Design review of the part built by this model. Coordinates are the model's own, in mm. Face numbers are marked on the shaded views. Coordinates: 2 decimals unless noted, no trailing zeros. Write each loop counter-clockwise with the first axis right and the second up, starting at its lowest first coordinate (ties: lowest second). Pieces come first, ordered by that corner, then holes.
```python
from build123d import *
from build123d.topology import SkipClean

# Parameters (mm, degrees)
SKETCH1_R           = 215.9
BOSS_EXTRUDE1_DEPTH = 50.8
SKETCH2_R           = 208.28
CUT_EXTRUDE1_DEPTH  = 43.18
CUT_EXTRUDE2_DEPTH  = 309.366879544
SKETCH4_R           = 5.715
CUT_EXTRUDE3_DEPTH  = 309.366879544


with BuildPart() as part:
    # Sketch1 → Boss-Extrude1 (new body)
    with BuildSketch(Plane(origin=(0, 0, 0), x_dir=(1, 0, 0), z_dir=(0, 1, 0))):
        with Locations(Location((0, 0, 0), (0, 0, 270))):
            Circle(SKETCH1_R)
    extrude(amount=BOSS_EXTRUDE1_DEPTH)

    # Sketch2 → Cut-Extrude1 (cut)
    with BuildSketch(Plane(origin=(0, 50.8, 0), x_dir=(1, 0, 0), z_dir=(0, 1, 0))):
        with Locations(Location((0, 0, 0), (0, 0, 270))):
            Circle(SKETCH2_R)
    extrude(amount=-CUT_EXTRUDE1_DEPTH, mode=Mode.SUBTRACT)

    # Sketch3 → Cut-Extrude2 (cut, through all)
    with SkipClean():  # the faces are left unmerged after this step: merging them gives an invalid solid
        with BuildSketch(Plane(origin=(0, 7.62, 0), x_dir=(1, 0, 0), z_dir=(0, 1, 0))):
            with BuildLine():
                Line((-63.5, -63.5), (63.5, -63.5))
                Line((63.5, -63.5), (63.5, -198.364080418))
                ThreePointArc((63.5, -198.364080418), (0, -208.28), (-63.5, -198.364080418))
                Line((-63.5, -198.364080418), (-63.5, -63.5))
            make_face()
        extrude(amount=-CUT_EXTRUDE2_DEPTH, mode=Mode.SUBTRACT)

    # Sketch4 → Cut-Extrude3 (cut, through all)
    with SkipClean():  # the faces are left unmerged after this step: merging them gives an invalid solid
        with BuildSketch(Plane(origin=(0, 7.62, 0), x_dir=(1, 0, 0), z_dir=(0, 1, 0))):
            with Locations(Location((0, 0, 0), (0, 0, 270))):
                Circle(SKETCH4_R)
        extrude(amount=-CUT_EXTRUDE3_DEPTH, mode=Mode.SUBTRACT)


solid = part.part
```
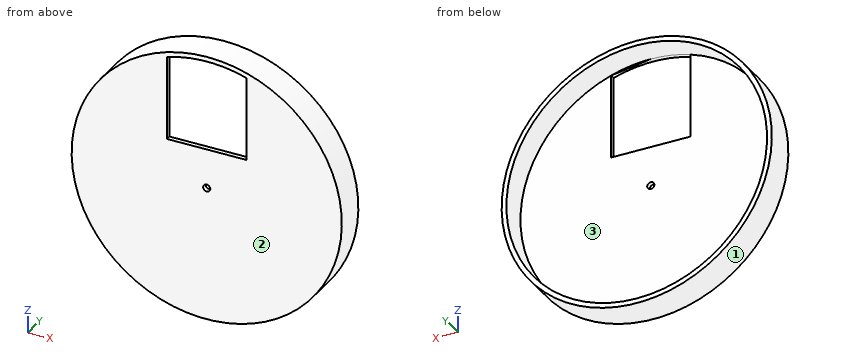
(1) Consider section B-B (z = -146). Give the boundary of the cut face in (x, y), plus the area to 3 significant figures.
(2) Insertion check: pin 1 Ø1 at (x, z) = (-60.5, -48) entering from +Y; pin 2 Ø4 at (x, y) = (78.5, 26.5) entering from +Z; pin 3 Ø4 at (x, y) = (35.5, 18) entering from -Z. Each pin has a flat end and moves straight along its axis. Give the tip position at first contact, or say it passes through.
(3) Consider section A-A (z = 0). Give the boundary of the cut face in (x, y) (3 decimals), plus the area to 3 significant figures.
(4) Consider section C-C (y = 36.5). Give the boundary of the cut face in (x, z).
(5) Mouldability with a two-part tool opening along X and no side actions: class the marked faces 1, 2 and 3 as +X half, -X half, draft (parallel to the pull), parting line (faces both ways), or undercut.
(6) Consider section D-D (z = 166). Give the boundary of the cut face in (x, y).
Results:
1. outline: (-159.05, 0) - (159.05, 0) - (159.05, 50.8) - (148.54, 50.8) - (148.54, 7.62) - (-148.54, 7.62) - (-148.54, 50.8) - (-159.05, 50.8) - close
1. area: 3,330 mm2
2. pin 1: stops at y = 7.62
2. pin 2: stops at z = 201.89
2. pin 3: stops at z = -213.29
3. outline: (-215.9, 0) - (-5.715, 0) - (-5.715, 7.62) - (-208.28, 7.62) - (-208.28, 50.8) - (-215.9, 50.8) - close; (5.715, 0) - (215.9, 0) - (215.9, 50.8) - (208.28, 50.8) - (208.28, 7.62) - (5.715, 7.62) - close
3. area: 3,860 mm2
4. outline: circle Ø431.8 at (0, 0); hole circle Ø416.56 at (0, 0)
5. face 1: parting line
5. face 2: draft
5. face 3: undercut
6. outline: (-138.05, 0) - (-63.5, 0) - (-63.5, 7.62) - (-125.8, 7.62) - (-125.8, 50.8) - (-138.05, 50.8) - close; (63.5, 0) - (138.05, 0) - (138.05, 50.8) - (125.8, 50.8) - (125.8, 7.62) - (63.5, 7.62) - close
